from build123d import *

# Parameters (mm, degrees)
F0_R     = 7.5
F1_DEPTH = 125
F2_R     = 15
F2_R_2   = 10.7
F3_DEPTH = 3.75


with BuildPart() as f1:
    # F0 (on Front) → F1 (new body)
    with BuildSketch(Plane.XZ):
        Circle(F0_R)
    extrude(amount=F1_DEPTH)

    # F2 (on Top) → F3 (join, symmetric)
    with BuildSketch(Plane.XY):
        with Locations((0, -136.475876)):
            Circle(F2_R)
        with Locations((0, -136.475876)):
            Circle(F2_R_2, mode=Mode.SUBTRACT)
    extrude(amount=F3_DEPTH, both=True)

    # F4: F1 across plane


with BuildPart() as f1_1:
    add(f1.part)
    add(f1.part.mirror(Plane.XZ))


solid = f1_1.part
Model file for the job. Use its own axes, mm. Round coordinates to 2 decimals unless told otherwise and drop trailing zeros. Order: outer loops, then holes, each group sorted by start corner. A loop starts at its lowest first (then second) coordinate and runs counter-clockwise, first axis right, second up. Notation, with made-up numbers: M 57.25,9 L 77.25,9 A20 ccw 77.25,19 Z; hole C 15,79 d11. An arc over 180 degrees is marked long. Write each question's results on one line, items separated by ' | '. Start each with the question number.
(1) Saw through at B-B, the plane z = 0. Give the cut face in (x, y).
(2) Saw through at A-A, the plane x = 0. Give the cut face in (y, z).
(3) Two-plate mould, pull along Y, no slides. Class faces 1 (the face through (-6, -146, 3.75)), 2 (the face through (-1.393, -125.867, -0.053)): pulls with the +Y half, pulls with the -Y half, needs draft (parallel to the pull), parting line crosses it, or undercut.
(4) Probe probe 1 along Y at (x, z) = (1, -2.5); probe 2 along Y at (x, z) = (0, -1.5); probe 3 along Y at (x, z) = (-2.5, 5.25). List the from-to ranges inside material, lowest first. Write a range as from..to.
(5) Saw through at C-C, the plane y = -86.5. Give the cut face in (x, z), then the cut area to 3 significant figures.
(6) Drop flat-ended pins along their axis: pin 1 (4 mm diameter, centred on x = -2.5, z = 5.5, fed in from +Y); pin 2 (1.5 mm diameter, centred on y = -120, z = -1, fed in from +X); pin 3 (1 mm diameter, centred on y = 118.5, z = -3, fed in from -X). Give the stop position or say it passes through.
Established:
1) outline: M -7.5,-123.49 A15 ccw long 7.5,-123.49 L 7.5,123.49 A15 ccw long -7.5,123.49 Z; hole C 0,-136.48 d21.4; hole C 0,136.48 d21.4
2) outline: M -151.48,-3.75 L -147.18,-3.75 L -147.18,3.75 L -151.48,3.75 Z; M -125.78,-3.75 L -125,-3.75 L -125,-7.5 L 125,-7.5 L 125,-3.75 L 125.78,-3.75 L 125.78,3.75 L 125,3.75 L 125,7.5 L -125,7.5 L -125,3.75 L -125.78,3.75 Z; M 147.18,-3.75 L 151.48,-3.75 L 151.48,3.75 L 147.18,3.75 Z
3) face 1: needs draft | face 2: undercut
4) probe 1: y = -151.44..-147.13, -125.82..125.82, 147.13..151.44 | probe 2: y = -151.48..-147.18, -125.78..125.78, 147.18..151.48 | probe 3: y = -125..125
5) outline: C 0,0 d15 | area: 177 mm^2
6) pin 1: stops at y = 151.4 | pin 2: stops at x = 7.5 | pin 3: stops at x = -7.07
